Drawing for the job (mm, zero at the part's lowest x, y, z). A direction names the side the tool comes from. Give positions to 0.01 mm unless a question says otherwise; leave off trailing zeros. Write each loop counter-clockwise with the first axis right and the second up, starting at its lowest first coordinate (ties: lowest second). Pieces come first, ordered by that corner, then holes. Notation, with made-up numbers: M -9.75,17 L 42.25,17 A27 ccw 42.25,38 Z; hole C 69,88.5 d2. An arc over 180 degrees is marked long. Use CSV: the item, a comma, the result in double quotes. Start each with the question number.
1. 3-axis set-ups, long thin cutter, end or side, ignore diameter. For the marked faces 1 and 2: which of +Z, -Z, +X, -X, +Y, -Y reach the whole face in a straight line?
2. Band-saw the part on B-B, the plane x = 6.35. List the corners of the cut face in (y, z) (3 decimals).
3. Band-saw the part on A-A, the plane z = 6.35. List the corners of the cut face in (x, y) (3 decimals), then the cut area to 3 significant figures.
4. Band-saw the part on D-D, the plane z = 1.5. List the corners of the cut face in (x, y) (3 decimals), then the cut area to 3 significant figures.
5. Drop flat-ended pins along their axis: pin 1 Ø1.5 at (x, y) = (8.5, 18.5) entering from -Z; pin 2 Ø3 at (y, z) = (4, 8.5) entering from -X; pin 3 Ø6.5 at (x, z) = (3.5, 3.5) entering from -Y. Give the stop position or say it passes through.
6. Mould opens along X. For the marked faces 3 and 4 say: pulls with the +X half, pulls with the -X half, needs draft (parallel to the pull), parting line crosses it, or undercut.
7. Band-saw the part on C-C, the plane y = 10.25. List the corners of the cut face in (x, z) (3 decimals).
8. Drill centre lines: line 1 along Y through (x, z) = (4, 11.5) (3 decimals); line 2 along X through (y, z) = (2, 9.5); line 3 along X through (y, z) = (22.5, 8.75). Where is each one in solid material? Low to high. Write a range as from..to.
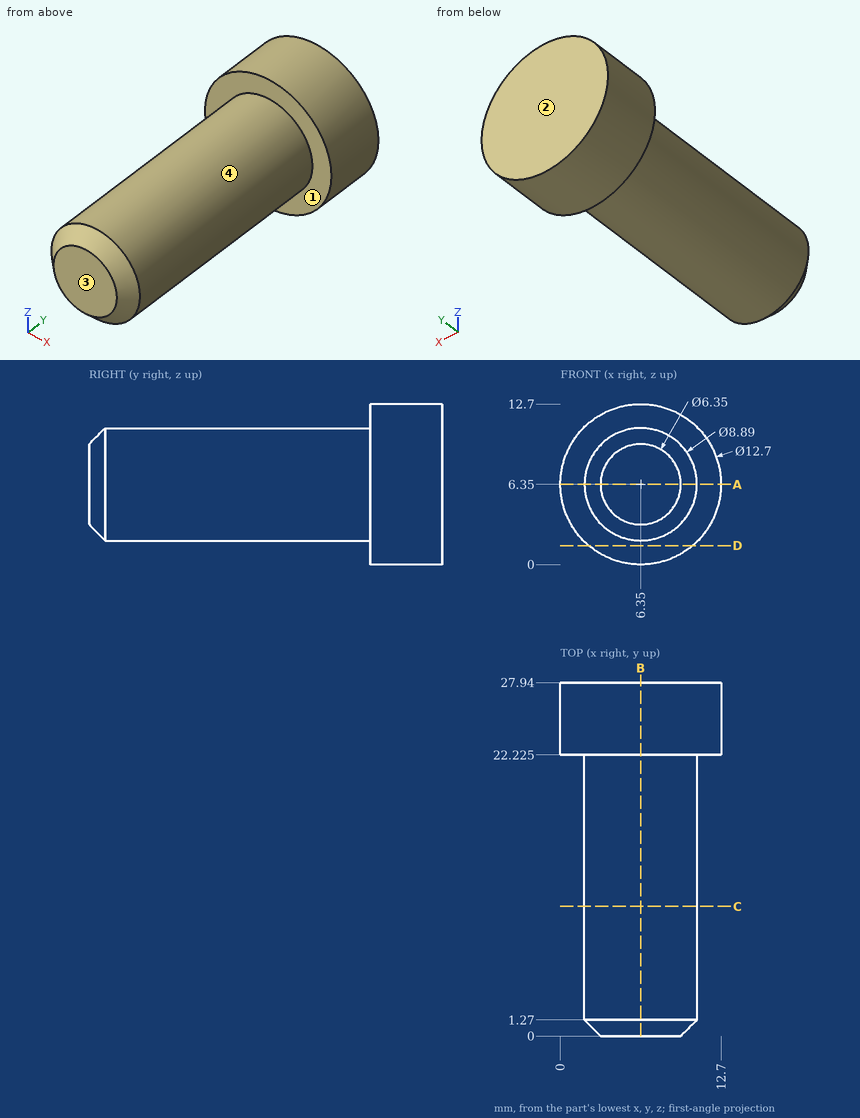
Output:
1,face 1,"-Y"
1,face 2,"+Z, -Z, +X, -X, +Y"
2,outline,"M 0,3.175 L 1.27,1.905 L 22.225,1.905 L 22.225,0 L 27.94,0 L 27.94,12.7 L 22.225,12.7 L 22.225,10.795 L 1.27,10.795 L 0,9.525 Z"
3,outline,"M 0,22.225 L 1.905,22.225 L 1.905,1.27 L 3.175,0 L 9.525,0 L 10.795,1.27 L 10.795,22.225 L 12.7,22.225 L 12.7,27.94 L 0,27.94 Z"
3,area,"269 mm²"
4,outline,"M 2.251,22.225 L 10.449,22.225 L 10.449,27.94 L 2.251,27.94 Z"
4,area,"46.8 mm²"
5,pin 1,"stops at z = 2.13"
5,pin 2,"stops at x = 1.95"
5,pin 3,"stops at y = 0"
6,face 3,"needs draft"
6,face 4,"parting line crosses it"
7,outline,"C 6.35,6.35 d8.89"
8,line 1,"y = 22.225..27.94"
8,line 2,"x = 3.21..9.49"
8,line 3,"x = 0.47..12.23"
